Source: CAD feature listing. Evaluate the final solid. Frame: model axes, mm. A direction names the side the tool comes from. Give positions to 0.01 mm unless a question says otherwise; leave off trailing zeros. Loops run counter-clockwise (first coordinate to the right, second up) from the corner with the lowest first, then second, coordinate; pieces in that order, holes last. Notation, with made-up numbers: M 16.5,20 L 56.5,20 A20 cw 56.5,44 Z; hole C -31,22 d11. An arc over 180 degrees is marked long. Answer in a Markdown table with one row per item.
Autodesk Inventor part; units mm, degrees
ref_plane "Arbeitsebene2" through (55.9, -6.9963, -17.125) normal (-1, 0, 0) x (0, 0, 1)
ref_plane "YZ Plane" through (0, 0, 0) normal (1, 0, 0) x (0, 1, 0)
ref_plane "XZ Plane" through (0, 0, 0) normal (0, 1, 0) x (-1, 0, 0)
ref_plane "Arbeitsebene1" through (0, 0, 0) normal (0, 0, 1) x (1, 0, 0)
sketch "Skizze1" plane through (0, 0, 0) normal (0, 0, 1) x (1, 0, 0)
  line L0 (8.6, 2.25) -> (8.6, -41.35)
  line L1 (8.6, -41.35) -> (-37.9, -41.35)
  line L2 (-37.9, -41.35) -> (-37.9, 2.25)
  line L3 (-37.9, 2.25) -> (8.6, 2.25)
  line L4 (9.6, 6.25) -> (-46.4, 6.25)
  line L5 (-46.4, 32.25) -> (-46.4, 6.25)
  line L6 (9.6, 32.25) -> (-46.4, 32.25)
  line L7 (9.6, 6.25) -> (9.6, 32.25)
  circle A0 centre (13.1, -11.2637) radius 1.4
  circle A1 centre (-42.4, -11.2637) radius 1.4
  circle A2 centre (-42.4, -31.25) radius 1.4
  line L8 (18.9, -41.35) -> (18.9, 19.75)
  line L9 (18.9, 19.75) -> (58.9, 19.75)
  line L10 (58.9, 19.75) -> (58.9, 19.25)
  line L11 (58.9, 19.25) -> (55.9, 19.25)
  line L12 (55.9, 17.6031) -> (55.9, 19.25)
  line L13 (63.9, 17.6031) -> (55.9, 17.6031)
  line L14 (63.9, 27.75) -> (63.9, 17.6031)
  arc A3 (63.9, 27.75) -> (58.9, 32.75) centre (58.9, 27.75) ccw
  line L15 (58.9, 32.75) -> (-58.9, 32.75)
  arc A4 (-58.9, 32.75) -> (-63.9, 27.75) centre (-58.9, 27.75) ccw
  line L16 (-63.9, -47.75) -> (-63.9, 27.75)
  arc A5 (-63.9, -47.75) -> (-58.9, -52.75) centre (-58.9, -47.75) ccw
  line L17 (-58.9, -52.75) -> (58.9, -52.75)
  arc A6 (58.9, -52.75) -> (63.9, -47.75) centre (58.9, -47.75) ccw
  line L18 (63.9, -47.75) -> (63.9, 0.8969)
  line L19 (55.9, 0.8969) -> (63.9, 0.8969)
  line L20 (55.9, -0.75) -> (55.9, 0.8969)
  line L21 (58.9, -0.75) -> (55.9, -0.75)
  line L22 (58.9, -0.75) -> (58.9, -1.25)
  line L23 (58.9, -1.25) -> (49.9, -1.25)
  line L24 (49.9, -1.25) -> (49.9, -41.35)
  line L25 (49.9, -41.35) -> (18.9, -41.35)
  circle A7 centre (13.1, 17.25) radius 1.4
  circle A8 centre (-50.2191, 17.25) radius 1.4
  line L26 (63.9, 17.6031) -> (63.9, 0.8969)
  line L27 (49.9, -1.25) -> (49.9, 19.75)
  line L28 (18.9, 6.25) -> (9.6, 6.25)
  line L29 (9.6, 6.25) -> (9.6, 2.25)
  line L30 (9.6, 2.25) -> (8.6, 2.25)
  line L31 (-37.9, 2.25) -> (-46.4, 2.25)
  line L32 (-46.4, 2.25) -> (-46.4, 6.25)
  line L33 (9.6, 32.25) -> (9.6, 32.75)
  line L34 (-46.4, 32.25) -> (-46.4, 32.75)
  circle A9 centre (58.9, 27.75) radius 1.4
  circle A10 centre (58.9, -47.75) radius 1.4
  circle A11 centre (-58.9, -47.75) radius 1.4
  circle A12 centre (-58.9, 27.75) radius 1.4
  line L35 (-46.4, 32.75) -> (9.6, 32.75)
  line L36 (9.6, 32.75) -> (9.6, 28.75)
  line L37 (9.6, 28.75) -> (-46.4, 28.75)
  line L38 (-46.4, 28.75) -> (-46.4, 32.75)
  point P0 (0, 0)
  point P1 (-46.4, 28.75)
  dimension "d0" = 2.8
  dimension "d1" = 2.8
  dimension "d2" = 2.8
  dimension "d3" = 2.8
  dimension "d29" = 4
extrude "Extrusion1" add sketch "Skizze1" along normal blind 5 contours L30 L29 L28 L8 L25 L24 L23 L22 L21 L20 L19 L18 A6 L17 A5 L16 A4 L15 L34 L5 L32 L31 L2 L1 L0 | L3 L31 L32 L4 L29 L30 | L7 L33 L15 A3 L14 L13 L12 L11 L10 L9 L8 L28 | L37 L5 L6 L7 | L6 L34 L15 L33 | L9 L10 L11 L12 L13 L26 L19 L20 L21 L22 L23 L27
sketch "Skizze3" plane through (0, 0, 5) normal (0, 0, 1) x (1, 0, 0)
  line L0 (-58.9, -52.75) -> (58.9, -52.75)
  arc A0 (58.9, -52.75) -> (63.9, -47.75) centre (58.9, -47.75) ccw
  line L1 (63.9, -47.75) -> (63.9, 27.75)
  arc A1 (63.9, 27.75) -> (58.9, 32.75) centre (58.9, 27.75) ccw
  line L2 (58.9, 32.75) -> (-58.9, 32.75)
  line L3 (9.6, 28.75) -> (9.6, 6.25)
  line L4 (9.6, 6.25) -> (-46.4, 6.25)
  line L5 (-46.4, 6.25) -> (-46.4, 28.75)
  arc A2 (-58.9, 32.75) -> (-63.9, 27.75) centre (-58.9, 27.75) ccw
  line L6 (-63.9, 27.75) -> (-63.9, -47.75)
  arc A3 (-63.9, -47.75) -> (-58.9, -52.75) centre (-58.9, -47.75) ccw
  circle A4 centre (13.1, 17.25) radius 1.4
  circle A5 centre (58.9, 27.75) radius 1.4
  circle A6 centre (13.1, -11.2637) radius 1.4
  circle A7 centre (-42.4, -11.2637) radius 1.4
  circle A8 centre (-42.4, -31.25) radius 1.4
  circle A9 centre (-50.2191, 17.25) radius 1.4
  circle A10 centre (-58.9, 27.75) radius 1.4
  circle A11 centre (-58.9, -47.75) radius 1.4
  circle A12 centre (58.9, -47.75) radius 1.4
  line L7 (8.6, 2.25) -> (8.6, -41.35)
  line L8 (8.6, -41.35) -> (-37.9, -41.35)
  line L9 (-37.9, -41.35) -> (-37.9, 2.25)
  line L10 (-37.9, 2.25) -> (8.6, 2.25)
  line L11 (18.9, -41.35) -> (18.9, 19.75)
  line L12 (18.9, 19.75) -> (49.9, 19.75)
  line L13 (49.9, 19.75) -> (49.9, -41.35)
  line L14 (49.9, -41.35) -> (18.9, -41.35)
  line L15 (-46.4, 28.75) -> (9.6, 28.75)
  point P0 (0, 0)
hole "Bohrung1" at (58.9, -47.75, 5) at (-58.9, -47.75, 5) at (-42.4, -31.25, 5) at (-42.4, -11.2637, 5) at (-50.2191, 17.25, 5) at (-58.9, 27.75, 5) at (13.1, -11.2637, 5) at (13.1, 17.25, 5) at (58.9, 27.75, 5) direction (0, 0, -1) diameter 2.9 end through all counterbore diameter 6.5 counterbore depth 3
ref_plane "Arbeitsebene2" through (55.9, -6.9963, -17.125) normal (-1, 0, 0) x (0, 0, 1)
sketch "Skizze7" plane through (0, 0, 5) normal (0, 0, 1) x (1, 0, 0)
  circle A0 centre (13.1, -11.2637) radius 3.25
  line L0 (18.9, -41.35) -> (18.9, 19.75)
  line L1 (18.9, 19.75) -> (49.9, 19.75)
  line L2 (49.9, 19.75) -> (49.9, -41.35)
  line L3 (49.9, -41.35) -> (18.9, -41.35)
  line L4 (-37.9, -41.35) -> (-37.9, 2.25)
  line L5 (-37.9, 2.25) -> (8.6, 2.25)
  line L6 (8.6, 2.25) -> (8.6, -41.35)
  circle A1 centre (13.1, 17.25) radius 3.25
  circle A2 centre (-58.9, 27.75) radius 3.25
  circle A3 centre (-42.4, -11.2637) radius 3.25
  circle A4 centre (-58.9, -47.75) radius 3.25
  circle A5 centre (58.9, -47.75) radius 3.25
  circle A6 centre (-42.4, -31.25) radius 3.25
  circle A7 centre (-50.2191, 17.25) radius 3.25
  circle A8 centre (58.9, 27.75) radius 3.25
  line L7 (58.9, 32.75) -> (-58.9, 32.75)
  arc A9 (-58.9, 32.75) -> (-63.9, 27.75) centre (-58.9, 27.75) ccw
  line L8 (-63.9, 27.75) -> (-63.9, -47.75)
  arc A10 (-63.9, -47.75) -> (-58.9, -52.75) centre (-58.9, -47.75) ccw
  line L9 (-58.9, -52.75) -> (58.9, -52.75)
  arc A11 (58.9, -52.75) -> (63.9, -47.75) centre (58.9, -47.75) ccw
  line L10 (63.9, -47.75) -> (63.9, 27.75)
  arc A12 (63.9, 27.75) -> (58.9, 32.75) centre (58.9, 27.75) ccw
  line L11 (9.6, 28.75) -> (9.6, 6.25)
  line L12 (9.6, 6.25) -> (-46.4, 6.25)
  line L13 (-46.4, 6.25) -> (-46.4, 28.75)
  line L14 (-46.4, 28.75) -> (9.6, 28.75)
  circle A13 centre (23.4151, 26.1333) radius 4
  circle A14 centre (46.9172, 26.1333) radius 4
  circle A15 centre (57.5383, 6.25) radius 4
  circle A16 centre (57.5383, -32.848) radius 4
  circle A17 centre (20.9293, -47.75) radius 4
  circle A18 centre (-29.9166, -47.75) radius 4
  circle A19 centre (-55.65, -19.55) radius 4
  line L15 (8.6, -41.35) -> (-37.9, -41.35)
  point P0 (0, 0)
  dimension "d33" = 8
  dimension "d34" = 8
  dimension "d35" = 8
  dimension "d36" = 8
  dimension "d37" = 8
  dimension "d38" = 8
  dimension "d39" = 8
extrude "Extrusion6" cut sketch "Skizze7" against normal blind 3.2 contours A13 | A14 | A15 | A16 | A17 | A18 | A19
properties part number "11_Wellplatespacer_magnetic"
1) Section A-A, the plane x = 31. Return loops of the section in (y, z), then the cut area to 3 significant figures.
Reply:
| item | result |
|---|---|
| outline | M -52.75,0 L -41.35,0 L -41.35,5 L -52.75,5 Z; M 19.75,0 L 32.75,0 L 32.75,5 L 19.75,5 Z |
| area | 122 mm² |
2) Section D-D, the plane y = 17.25. Return loops of the section in (x, z).
Reply:
| item | result |
|---|---|
| outline | M -63.9,0 L -51.67,0 L -51.67,2 L -53.47,2 L -53.47,5 L -63.9,5 Z; M -48.77,0 L -46.4,0 L -46.4,5 L -46.97,5 L -46.97,2 L -48.77,2 Z; M 9.6,0 L 11.65,0 L 11.65,2 L 9.85,2 L 9.85,5 L 9.6,5 Z; M 14.55,0 L 18.9,0 L 18.9,5 L 16.35,5 L 16.35,2 L 14.55,2 Z; M 49.9,0 L 63.9,0 L 63.9,5 L 49.9,5 Z |
3) Section B-B, the plane y = -19.55. Return loops of the section in (x, z), then the cut area to 3 significant figures.
Reply:
| item | result |
|---|---|
| outline | M -63.9,0 L -37.9,0 L -37.9,5 L -51.65,5 L -51.65,1.8 L -59.65,1.8 L -59.65,5 L -63.9,5 Z; M 8.6,0 L 18.9,0 L 18.9,5 L 8.6,5 Z; M 49.9,0 L 63.9,0 L 63.9,5 L 49.9,5 Z |
| area | 226 mm² |
4) Set-up query: faces 1 (the flat face through (-15, 2.25, 2)), 2 (the cylindrical face through (43.74, 23.7, 3.42)), 3 (the cylindrical face through (62.47, -51.25, 2.46)). Return all of +Z, -Z, +X, -X, +Y, -Y with unobstructed straight access to the full face (end or side cutting, diameter ignored); none if empty.
Reply:
| item | result |
|---|---|
| face 1 | +Z, -Z |
| face 2 | +Z |
| face 3 | +Z, -Z, +X, -Y |
5) Section C-C, the plane x = -13. Return loops of the section in (y, z), then the cut area to 3 significant figures.
Reply:
| item | result |
|---|---|
| outline | M -52.75,0 L -41.35,0 L -41.35,5 L -52.75,5 Z; M 2.25,0 L 6.25,0 L 6.25,5 L 2.25,5 Z; M 28.75,0 L 32.75,0 L 32.75,5 L 28.75,5 Z |
| area | 97.0 mm² |
6) Pull-direction query (X, two-part tool) for faces 4 (the flat face through (-18, 28.75, 2)), 5 (the flat face through (-59, -46, 2)), 6 (the cylindrical face through (-62.4, -51.32, 2.46)), 7 (the flat face through (-1, -52.75, 2)); classes: released by +X, released by -X, zero draft, split by the parting line, or undercut.
Reply:
| item | result |
|---|---|
| face 4 | undercut |
| face 5 | undercut |
| face 6 | released by -X |
| face 7 | zero draft |
7) Pin query (flat end, axial travel): pin 1 Ø5 at (x, y) = (12.5, -10) entering from +Z; pin 2 Ø2 at (x, y) = (-59, 28.5) entering from +Z; pin 3 Ø6.5 at (x, y) = (-29.92, -47.75) entering from +Z. Return the tip coordinate at first contact, or that it passes through.
Reply:
| item | result |
|---|---|
| pin 1 | stops at z = 5 |
| pin 2 | stops at z = 2 |
| pin 3 | stops at z = 1.8 |
8) Material intervals for L1, parallel to Y at x = -42.4, z = 0.8; L2, parallel to X at y = 17.25, z = 2.85; L3, parallel to X at y = 6.5, z = 3.7, sorted ascending.
Reply:
| item | result |
|---|---|
| L1 | y = -52.75 to -32.7, -29.8 to -12.71, -9.81 to 6.25, 28.75 to 32.75 |
| L2 | x = -63.9 to -53.47, -46.97 to -46.4, 9.6 to 9.85, 16.35 to 18.9, 49.9 to 63.9 |
| L3 | x = -63.9 to -46.4, 9.6 to 18.9, 49.9 to 53.55, 61.53 to 63.9 |
